Geometry check sheet. Reference: the model listing, model coordinates, mm. Round coordinates to 2 decimals unless told otherwise and drop trailing zeros. Loops run counter-clockwise (first coordinate to the right, second up) from the corner with the lowest first, then second, coordinate; pieces in that order, holes last. Notation, with made-up numbers: M 87,40.5 L 98,40.5 A24 ccw 98,65.5 Z; hole C 24,12.5 d11. An arc over 180 degrees is marked long. Use one line per item in the form item = value. Start each with the question number.
1. Cross-section at B-B (x = -29). Record the boundary of the cut face in (y, z), then the cut area to 3 significant figures.
2. Cross-section at D-D (y = 0.85). Record the boundary of the cut face in (x, z), then the cut area to 3 significant figures.
3. Draft check along X on faces 1 (the flat face through (-2, 0, -2)), 2 (the cylindrical face through (149.474, 1.014, -68.268)), 3 (the cylindrical face through (-14.335, 1.014, -68.268)). Enter one of: pulls with the +X half, pulls with the -X half, needs draft (parallel to the pull), parting line crosses it, or undercut.
4. Cross-section at C-C (z = -9). Record the boundary of the cut face in (x, y), then the cut area to 3 significant figures.
5. Cross-section at A-A (z = -73). Record the boundary of the cut face in (x, y).
6. Material ranges on line 1 (X direction, y = 1.65, z = -66.5); line 2 (X direction, y = 0.1, z = -48); line 3 (Z direction, x = 131.5, y = 0.25), recorded low to high.
```python
from build123d import *

# Parameters (mm, degrees)
SKETCH1_W           = 325
SKETCH1_H           = 250
BOSS_EXTRUDE1_DEPTH = 2
CUT_EXTRUDE1_REACH  = 4
SKETCH2_R           = 16.5


with BuildPart() as part:
    # Sketch1 → Boss-Extrude1 (new body)
    with BuildSketch(Plane(origin=(0, 0, 0), x_dir=(1, 0, 0), z_dir=(0, 1, 0))):
        Rectangle(SKETCH1_W, SKETCH1_H)
    extrude(amount=BOSS_EXTRUDE1_DEPTH)

    # Sketch2 → Cut-Extrude1 (cut, up to next)
    with BuildSketch(Plane(origin=(0, 2, 0), x_dir=(1, 0, 0), z_dir=(0, 1, 0)), mode=Mode.PRIVATE) as cut_extrude1_sk1:
        with Locations((133.736379862, 1.843557571)):
            Circle(SKETCH2_R)
    cut_extrude1_tool1 = extrude(cut_extrude1_sk1.sketch, amount=-CUT_EXTRUDE1_REACH, mode=Mode.PRIVATE) & part.part
    add(cut_extrude1_tool1.solids().sort_by_distance((133.73638, 2, -1.843558))[0], mode=Mode.SUBTRACT)
    # Sketch2 → Cut-Extrude1 (cut, up to next)
    with BuildSketch(Plane(origin=(0, 2, 0), x_dir=(1, 0, 0), z_dir=(0, 1, 0)), mode=Mode.PRIVATE) as cut_extrude1_sk2:
        with Locations((133.736379862, 63.311910549)):
            Circle(SKETCH2_R)
    cut_extrude1_tool2 = extrude(cut_extrude1_sk2.sketch, amount=-CUT_EXTRUDE1_REACH, mode=Mode.PRIVATE) & part.part
    add(cut_extrude1_tool2.solids().sort_by_distance((133.73638, 2, -63.311911))[0], mode=Mode.SUBTRACT)
    # Sketch2 → Cut-Extrude1 (cut, up to next)
    with BuildSketch(Plane(origin=(0, 2, 0), x_dir=(1, 0, 0), z_dir=(0, 1, 0)), mode=Mode.PRIVATE) as cut_extrude1_sk3:
        with Locations((-30.073468299, 63.311910549)):
            Circle(SKETCH2_R)
    cut_extrude1_tool3 = extrude(cut_extrude1_sk3.sketch, amount=-CUT_EXTRUDE1_REACH, mode=Mode.PRIVATE) & part.part
    add(cut_extrude1_tool3.solids().sort_by_distance((-30.073468, 2, -63.311911))[0], mode=Mode.SUBTRACT)


solid = part.part
```
Reported:
q1.outline = M 0,-125 L 2,-125 L 2,-79.78 L 0,-79.78 Z; M 0,-46.85 L 2,-46.85 L 2,125 L 0,125 Z
q1.area = 434 mm²
q2.outline = M -162.5,-125 L 162.5,-125 L 162.5,125 L -162.5,125 Z; hole C -30.07,-63.31 d33; hole C 133.74,-63.31 d33; hole C 133.74,-1.84 d33
q2.area = 78,700 mm²
q3.face_1 = needs draft
q3.face_2 = undercut
q3.face_3 = undercut
q4.outline = M -162.5,0 L 118.87,0 L 118.87,2 L -162.5,2 Z; M 148.6,0 L 162.5,0 L 162.5,2 L 148.6,2 Z
q4.area = 591 mm²
q5.outline = M -162.5,0 L -43.43,0 L -43.43,2 L -162.5,2 Z; M -16.72,0 L 120.38,0 L 120.38,2 L -16.72,2 Z; M 147.09,0 L 162.5,0 L 162.5,2 L 147.09,2 Z
q6.line_1 = -162.5 to -46.26, -13.88 to 117.55, 149.93 to 162.5
q6.line_2 = -162.5 to -36.22, -23.93 to 127.59, 139.88 to 162.5
q6.line_3 = -125 to -79.66, -46.96 to -18.19, 14.5 to 125
